Geometry: final body of the model. Coordinates: model frame, mm. Face numbers are marked on the shaded views. A direction names the side the tool comes from. Give positions to 0.01 mm unless a question says otherwise; leave off trailing zeros. Write each loop counter-clockwise with the first axis right and the second up, starting at its lowest first coordinate (ties: lowest second). Pieces come first, ordered by that corner, then holes. Notation, with made-up numbers: (18, 59.25) -> (34, 59.25) arc R26 cw to (34, 98.25) -> close; hole circle Ø8 at (21.25, 56.5). An arc over 180 degrees is marked (long way). Answer as a JSON object with one key per item and string values.
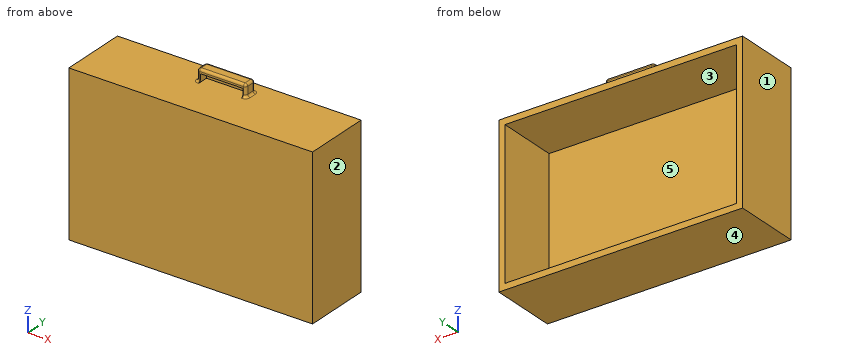
from build123d import *

# Parameters (mm, degrees)
SKETCH2_W           = 254
SKETCH2_H           = 165.1
BOSS_EXTRUDE1_DEPTH = 6.35
SKETCH3_W           = 254
SKETCH3_H           = 165.1
SKETCH3_W_2         = 241.3
SKETCH3_H_2         = 152.4
BOSS_EXTRUDE2_DEPTH = 63.5
SKETCH4_W           = 50.8
SKETCH4_H           = 12.7
BOSS_EXTRUDE3_DEPTH = 12.7
SKETCH6_W           = 44.45
SKETCH6_H           = 8.276182153
CUT_EXTRUDE1_DEPTH  = 8.89
FILLET1_R           = 2.54


with BuildPart() as part:
    # Sketch2 → Boss-Extrude1 (new body)
    with BuildSketch(Plane(origin=(0, 0, 0), x_dir=(1, 0, 0), z_dir=(0, 1, 0))):
        Rectangle(SKETCH2_W, SKETCH2_H)
    extrude(amount=BOSS_EXTRUDE1_DEPTH)

    # Sketch3 → Boss-Extrude2 (add)
    with BuildSketch(Plane(origin=(0, 6.35, 0), x_dir=(1, 0, 0), z_dir=(0, 1, 0))):
        Rectangle(SKETCH3_W, SKETCH3_H)
        Rectangle(SKETCH3_W_2, SKETCH3_H_2, mode=Mode.SUBTRACT)
    extrude(amount=BOSS_EXTRUDE2_DEPTH)

    # Sketch4 → Boss-Extrude3 (add)
    with BuildSketch(Plane.XY.offset(82.55)):
        with Locations((0, 50.8)):
            Rectangle(SKETCH4_W, SKETCH4_H)
    extrude(amount=BOSS_EXTRUDE3_DEPTH)

    # Sketch6 → Cut-Extrude1 (cut)
    with BuildSketch(Plane(origin=(0, 44.45, 0), x_dir=(-1, 0, 0), z_dir=(0, -1, 0))):
        with Locations((0, -86.688091077)):
            Rectangle(SKETCH6_W, SKETCH6_H)
    extrude(amount=-CUT_EXTRUDE1_DEPTH, mode=Mode.SUBTRACT)

    # Fillet1
    fillet1_edges = [part.edges().sort_by_distance(p)[0] for p in [
        (-25.4, 50.8, 82.55),
        (-25.4, 57.15, 88.9),
        (-23.8125, 44.45, 82.55),
        (-25.4, 44.45, 88.9),
        (25.4, 50.8, 82.55),
        (25.4, 44.45, 88.9),
        (0, 57.15, 82.55),
        (25.4, 57.15, 88.9),
        (-25.4, 50.8, 95.25),
        (0, 44.45, 95.25),
        (25.4, 50.8, 95.25),
        (0, 57.15, 95.25),
        (23.8125, 44.45, 82.55),
    ]]
    fillet(fillet1_edges, radius=FILLET1_R)


solid = part.part
Q1. Mould query, pull axis X, two halves, no side actions, for the marked faces 1, 2 and 3. Classes: pulls with the +X half, pulls with the -X half, needs draft (parallel to the pull), parting line crosses it, or undercut.
Values:
{"face 1": "pulls with the -X half", "face 2": "pulls with the +X half", "face 3": "undercut"}
Q2. Cut plane D-D (y = 35.5). Return the cut outline in (x, z), and give its area (3 significant figures).
Values:
{"outline": "(-127, -82.55) -> (127, -82.55) -> (127, 82.55) -> (-127, 82.55) -> close; hole (-120.65, -76.2) -> (120.65, -76.2) -> (120.65, 76.2) -> (-120.65, 76.2) -> close", "area": "5,160 mm²"}
Q3. First-contact query: P1, Ø4, axis at x = 4, z = 89, coming from the -Y side; P2, Ø10, axis at x = -44.5, y = 25, coming from the +Z side; P3, Ø6, axis at y = 49, z = 88, coming from the +X side. Flat tips, straight axial feed; report the tip coordinate or a pass-through.
Values:
{"P1": "y = 44.45", "P2": "z = 82.55", "P3": "x = 25.4"}
Q4. Cut plane C-C (z = 35). Return the cut outline in (x, y).
Values:
{"outline": "(-127, 0) -> (127, 0) -> (127, 69.85) -> (120.65, 69.85) -> (120.65, 6.35) -> (-120.65, 6.35) -> (-120.65, 69.85) -> (-127, 69.85) -> close"}
Q5. Material intervals for L1, parallel to X at y = 61.5, z = 59.5; L2, parallel to Z at x = -108, y = 36; L3, parallel to Y at x = -59, z = 65, sorted ascending. Write a range as from..to.
Values:
{"L1": "-127..-120.65, 120.65..127", "L2": "-82.55..-76.2, 76.2..82.55", "L3": "0..6.35"}
Q6. Cut plane B-B (x = -85.5). Return the cut outline in (y, z).
Values:
{"outline": "(0, -82.55) -> (69.85, -82.55) -> (69.85, -76.2) -> (6.35, -76.2) -> (6.35, 76.2) -> (69.85, 76.2) -> (69.85, 82.55) -> (0, 82.55) -> close"}
Q7. Set-up query: the marked faces 4 and 5. Return all of +Z, -Z, +X, -X, +Y, -Y with unobstructed straight access to the full face (end or side cutting, diameter ignored); none if empty.
Values:
{"face 4": "-Z, +X, -X, +Y, -Y", "face 5": "+Y"}
Q8. Cut plane A-A (y = 50). Return the cut outline in (x, z) (3 decimals).
Values:
{"outline": "(-127, -82.55) -> (127, -82.55) -> (127, 82.55) -> (27.94, 82.55) arc R2.54 cw to (25.4, 85.09) -> (25.4, 92.71) arc R2.54 ccw to (22.86, 95.25) -> (-22.86, 95.25) arc R2.54 ccw to (-25.4, 92.71) -> (-25.4, 85.09) arc R2.54 cw to (-27.94, 82.55) -> (-127, 82.55) -> close; hole (-120.65, -76.2) -> (120.65, -76.2) -> (120.65, 76.2) -> (-120.65, 76.2) -> close; hole (-22.225, 82.55) -> (22.225, 82.55) -> (22.225, 90.826) -> (-22.225, 90.826) -> close"}
